```python
from build123d import *

# Parameters (mm, degrees)
SKIZZE1_W                       = 42
SKIZZE1_H                       = 63
SKIZZE1_R                       = 18.1
SKIZZE1_R_2                     = 1.7
SKIZZE1_R_3                     = 2.3
AUFSATZ_LINEAR_AUSTRAGEN1_DEPTH = 13
SKIZZE2_W                       = 42
SKIZZE2_H                       = 42
SKIZZE2_R                       = 18.1
SKIZZE2_R_2                     = 1.7
AUFSATZ_LINEAR_AUSTRAGEN2_DEPTH = 20
SKIZZE4_R                       = 4
SCHNITT_LINEAR_AUSTRAGEN1_DEPTH = 10
SKIZZE5_R                       = 2.9
SCHNITT_LINEAR_AUSTRAGEN2_DEPTH = 30
FASE1_SIZE                      = 3
FASE2_SIZE                      = 8


with BuildPart() as part:
    # Skizze1 → Aufsatz-Linear austragen1 (new body)
    with BuildSketch(Plane.XY):
        with Locations((0, -10.5)):
            Rectangle(SKIZZE1_W, SKIZZE1_H)
        Circle(SKIZZE1_R, mode=Mode.SUBTRACT)
        with Locations((-15.5, 15.5)):
            Circle(SKIZZE1_R_2, mode=Mode.SUBTRACT)
        with Locations((15.5, 15.5)):
            Circle(SKIZZE1_R_2, mode=Mode.SUBTRACT)
        with Locations((-15.5, -15.5)):
            Circle(SKIZZE1_R_2, mode=Mode.SUBTRACT)
        with Locations((15.5, -15.5)):
            Circle(SKIZZE1_R_2, mode=Mode.SUBTRACT)
        with Locations((-15.5, -32)):
            Circle(SKIZZE1_R_3, mode=Mode.SUBTRACT)
        with Locations((15.5, -32)):
            Circle(SKIZZE1_R_3, mode=Mode.SUBTRACT)
    extrude(amount=AUFSATZ_LINEAR_AUSTRAGEN1_DEPTH)

    # Skizze2 → Aufsatz-Linear austragen2 (add)
    with BuildSketch(Plane.XY.offset(13)):
        Rectangle(SKIZZE2_W, SKIZZE2_H)
        Circle(SKIZZE2_R, mode=Mode.SUBTRACT)
        with Locations((15.5, 15.5)):
            Circle(SKIZZE2_R_2, mode=Mode.SUBTRACT)
        with Locations((15.5, -15.5)):
            Circle(SKIZZE2_R_2, mode=Mode.SUBTRACT)
        with Locations((-15.5, -15.5)):
            Circle(SKIZZE2_R_2, mode=Mode.SUBTRACT)
        with Locations((-15.5, 15.5)):
            Circle(SKIZZE2_R_2, mode=Mode.SUBTRACT)
    extrude(amount=AUFSATZ_LINEAR_AUSTRAGEN2_DEPTH)

    # Skizze4 → Schnitt-Linear austragen1 (cut)
    with BuildSketch(Plane.XY):
        with Locations((-15.5, -32)):
            Circle(SKIZZE4_R)
        with Locations((15.5, -32)):
            Circle(SKIZZE4_R)
    extrude(amount=SCHNITT_LINEAR_AUSTRAGEN1_DEPTH, mode=Mode.SUBTRACT)

    # Skizze5 → Schnitt-Linear austragen2 (cut)
    with BuildSketch(Plane.XY):
        with Locations((-15.5, 15.5)):
            Circle(SKIZZE5_R)
        with Locations((15.5, 15.5)):
            Circle(SKIZZE5_R)
        with Locations((-15.5, -15.5)):
            Circle(SKIZZE5_R)
        with Locations((15.5, -15.5)):
            Circle(SKIZZE5_R)
    extrude(amount=SCHNITT_LINEAR_AUSTRAGEN2_DEPTH, mode=Mode.SUBTRACT)

    # Fase1
    fase1_edges = [part.edges().sort_by_distance(p)[0] for p in [
        (-21, -21, 23),
        (21, -21, 23),
        (-21, 21, 16.5),
        (21, 21, 16.5),
    ]]
    chamfer(fase1_edges, length=FASE1_SIZE)

    # Fase2
    fase2_edges = [part.edges().sort_by_distance(p)[0] for p in [
        (21, -42, 6.5),
        (-21, -42, 6.5),
    ]]
    chamfer(fase2_edges, length=FASE2_SIZE)


solid = part.part
```
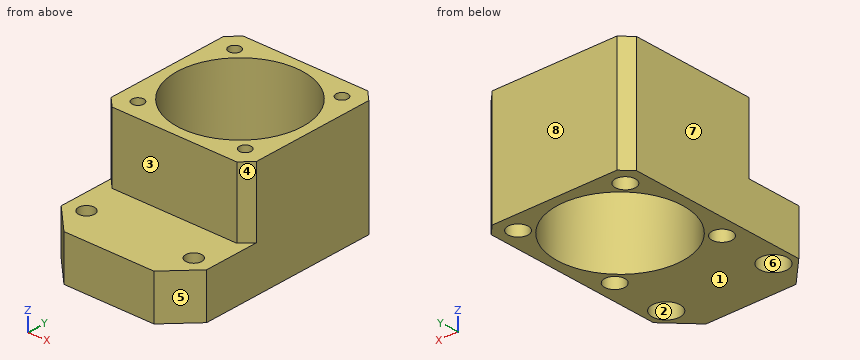
Design review of the part built by this model. Coordinates are the model's own, in mm. Face numbers are marked on the shaded views. A direction names the side the tool comes from. Coordinates: 2 decimals unless noted, no trailing zeros. Loops run counter-clockwise (first coordinate to the right, second up) from the corner with the lowest first, then second, coordinate; pieces in that order, holes last.
Q1. Tool access review of the marked faces 1, 2, 3, 4 and 5: name each direction out of +Z, -Z, +X, -X, +Y, -Y from which nothing blocks a thin tool from reaching the whole face with its end or side.
Reported:
face 1: -Z, +X, -X, +Y, -Y
face 2: -Z
face 3: +Z, +X, -X, -Y
face 4: +Z, +X, -Y
face 5: +Z, -Z, +X, -Y
Q2. We need section D-D on z = 12. State the section outline as (x, y) points.
Reported:
outline: (-21, -34) - (-13, -42) - (13, -42) - (21, -34) - (21, 18) - (18, 21) - (-18, 21) - (-21, 18) - close; hole circle Ø5.8 at (-15.5, -15.5); hole circle Ø5.8 at (-15.5, 15.5); hole circle Ø36.2 at (0, 0); hole circle Ø4.6 at (-15.5, -32); hole circle Ø5.8 at (15.5, -15.5); hole circle Ø5.8 at (15.5, 15.5); hole circle Ø4.6 at (15.5, -32)
Q3. The part is to be moulded in two halves that separate along Y. For the marked faces 6, 7 and 8, say which applies: +Y half, -Y half, draft (parallel to the pull), parting line (faces both ways), or undercut.
Reported:
face 6: undercut
face 7: draft
face 8: +Y half
Q4. For pin 1 (2.5 mm diameter, centred on x = 14, y = -30.5, fed in from -Z); pin 2 (4 mm diameter, centred on x = 15.5, y = -15.5, fed in from -Z), all flat-tipped, find the tip position at first contact; note any pin that passes through.
Reported:
pin 1: stops at z = 10
pin 2: stops at z = 30
Q5. We need section B-B on x = 0. State the section outline as (y, z) points.
Reported:
outline: (-42, 0) - (-18.1, 0) - (-18.1, 33) - (-21, 33) - (-21, 13) - (-42, 13) - close; (18.1, 0) - (21, 0) - (21, 33) - (18.1, 33) - close
Q6. To check wall thickness, follow line 1 (X direction, y = -15.5, z = 31.45); line 2 (X direction, y = 14, z = 30.5); line 3 (Y direction, x = 15.5, z = 7.75). State the ranges of each line that lie inside material, in increasing order.
Reported:
line 1: x = -21 to -17.2, -13.8 to -9.35, 9.35 to 13.8, 17.2 to 21
line 2: x = -21 to -16.3, -14.7 to -11.47, 11.47 to 14.7, 16.3 to 21
line 3: y = -39.5 to -36, -28 to -18.4, -12.6 to -9.35, 9.35 to 12.6, 18.4 to 21
Q7. We need section C-C on z = 24.5. State the section outline as (x, y) points.
Reported:
outline: (-21, -18) - (-18, -21) - (18, -21) - (21, -18) - (21, 18) - (18, 21) - (-18, 21) - (-21, 18) - close; hole circle Ø5.8 at (-15.5, -15.5); hole circle Ø5.8 at (-15.5, 15.5); hole circle Ø36.2 at (0, 0); hole circle Ø5.8 at (15.5, -15.5); hole circle Ø5.8 at (15.5, 15.5)
Q8. We need section A-A on y = 0. State the section outline as (x, z) points, and give its area (3 significant figures).
Reported:
outline: (-21, 0) - (-18.1, 0) - (-18.1, 33) - (-21, 33) - close; (18.1, 0) - (21, 0) - (21, 33) - (18.1, 33) - close
area: 191 mm2
